from build123d import *

# Parameters (mm, degrees)
SKETCH1_W               = 140
SKETCH1_H               = 90
BOSS_EXTRUDE1_DEPTH     = 42
CUT_EXTRUDE1_DEPTH      = 30
FILLET2_R               = 3
SKETCH3_W               = 140
SKETCH3_H               = 60
BOSS_EXTRUDE2_DEPTH     = 5
SKETCH4_W               = 3
SKETCH4_H               = 60
BOSS_EXTRUDE3_DEPTH     = 19
CUT_EXTRUDE2_DEPTH      = 172.650808329
CUT_EXTRUDE2_DEPTH_BACK = 172.650808329


with BuildPart() as part:
    # Sketch1 → Boss-Extrude1 (new body)
    with BuildSketch(Plane(origin=(0, 0, 0), x_dir=(1, 0, 0), z_dir=(0, 1, 0))):
        with Locations((70, 45)):
            Rectangle(SKETCH1_W, SKETCH1_H)
    extrude(amount=BOSS_EXTRUDE1_DEPTH)

    # Sketch2 → Cut-Extrude1 (cut)
    with BuildSketch(Plane(origin=(0, 42, 0), x_dir=(1, 0, 0), z_dir=(0, 1, 0))):
        Polygon((7.5, 8), (7.5, 83), (62.5, 83), (62.5, 8), (45, 8), (45, 0), (25, 0), (25, 8), align=None)
        Polygon((77.5, 8), (77.5, 83), (132.5, 83), (132.5, 8), (115, 8), (115, 0), (95, 0), (95, 8), align=None)
    extrude(amount=-CUT_EXTRUDE1_DEPTH, mode=Mode.SUBTRACT)

    # Fillet2
    fillet2_edges = [part.edges().sort_by_distance(p)[0] for p in [
        (140, 42, -45),
        (70, 42, 0),
        (127.5, 42, 0),
        (70, 42, -90),
        (25, 27, -8),
        (45, 27, -8),
        (45, 27, 0),
        (25, 27, 0),
        (25, 42, -4),
        (45, 42, -4),
        (95, 27, -8),
        (115, 27, -8),
        (115, 27, 0),
        (95, 27, 0),
        (95, 42, -4),
        (115, 42, -4),
        (0, 42, -45),
        (70, 0, -90),
        (0, 21, -90),
        (140, 21, -90),
        (12.5, 42, 0),
    ]]
    fillet(fillet2_edges, radius=FILLET2_R)

    # Sketch3 → Boss-Extrude2 (add)
    with BuildSketch(Plane(origin=(0, 0, 0), x_dir=(1, 0, 0), z_dir=(0, 1, 0))):
        with Locations((70, -30)):
            Rectangle(SKETCH3_W, SKETCH3_H)
    extrude(amount=BOSS_EXTRUDE2_DEPTH)

    # Sketch4 → Boss-Extrude3 (add)
    with BuildSketch(Plane(origin=(0, 5, 0), x_dir=(1, 0, 0), z_dir=(0, 1, 0))):
        with Locations((1.5, -30)):
            Rectangle(SKETCH4_W, SKETCH4_H)
        with Locations((138.5, -30)):
            Rectangle(SKETCH4_W, SKETCH4_H)
    extrude(amount=BOSS_EXTRUDE3_DEPTH)

    # Sketch5 → Cut-Extrude2 (cut, two sides: drawn at the far end of the back side and taken through both)
    with BuildSketch(Plane.ZY.offset(-CUT_EXTRUDE2_DEPTH_BACK)):
        Polygon((60, 0), (8.038475773, 30), (60, 30), align=None)
    extrude(amount=CUT_EXTRUDE2_DEPTH + CUT_EXTRUDE2_DEPTH_BACK, mode=Mode.SUBTRACT)


solid = part.part
Model file for the job. Use its own axes, mm. A direction names the side the tool comes from. Round coordinates to 2 decimals unless told otherwise and drop trailing zeros. Loops run counter-clockwise (first coordinate to the right, second up) from the corner with the lowest first, then second, coordinate; pieces in that order, holes last.
1. Mould opens along Z. For faces 4 (the flat face through (70.327, 4.833, 51.629)), 5 (the flat face through (137, 12, 20)), 6 (the flat face through (55, 27, -8)) say: +Z half, -Z half, draft (parallel to the pull), parting line (faces both ways), or undercut.
Check values:
face 4: +Z half
face 5: draft
face 6: undercut
2. Tool access for faces 1 (the flat face through (3, 12, 20)), 2 (the flat face through (70, 42, -48)), 3 (the flat face through (35, 12, -42)): list every direction of +Z, -Z, +X, -X, +Y, -Y with a clear straight run to the whole face (end or side of a thin tool).
Check values:
face 1: +Z, +Y
face 2: +Z, -Z, +X, -X, +Y
face 3: +Y
3. Wall check: probe 1 along X at (y, z) = (15.5, -10.5); probe 2 along Z at (x, y) = (132, 19); probe 3 along Y at (x, z) = (29, -70). Give the ranges that are in metal, low to high.
Check values:
probe 1: x = 0 to 7.5, 62.5 to 77.5, 132.5 to 140
probe 2: z = -90 to -83, -8 to 0
probe 3: y = 0 to 12
4. Band-saw the part on D-D, the plane x = 75. List the corners of the cut face in (y, z), and give its area (3 significant figures).
Check values:
outline: (0, -87) arc R3 ccw to (3, -90) - (39, -90) arc R3 ccw to (42, -87) - (42, -3) arc R3 ccw to (39, 0) - (5, 0) - (5, 51.34) - (0, 60) - close
area: 4,050 mm2
5. Band-saw the part on C-C, the plane z = -33.5. List the corners of the cut face in (x, y).
Check values:
outline: (0, 0) - (140, 0) - (140, 39) arc R3 ccw to (137, 42) - (132.5, 42) - (132.5, 12) - (77.5, 12) - (77.5, 42) - (62.5, 42) - (62.5, 12) - (7.5, 12) - (7.5, 42) - (3, 42) arc R3 ccw to (0, 39) - close
6. Drop flat-ended pins along their axis: P1, Ø9, axis at x = 44, y = 23, coming from the +Z side; P2, Ø16.5, axis at x = 31.5, z = -42, coming from the +Y side; P3, Ø3, axis at x = 76.5, y = 6, coming from the +Z side; P4, Ø10, axis at y = 30.5, z = 13, coming from the +X side. Give the stop position or say it passes through.
Check values:
P1: stops at z = 0
P2: stops at y = 12
P3: stops at z = 52.21
P4: passes through
7. Band-saw the part on B-B, the plane x = 100. List the corners of the cut face in (y, z).
Check values:
outline: (0, -87) arc R3 ccw to (3, -90) - (39, -90) arc R3 ccw to (42, -87) - (42, -83) - (12, -83) - (12, 0) - (5, 0) - (5, 51.34) - (0, 60) - close
